Design review of the part built by this model. Coordinates are the model's own, in mm. A direction names the side the tool comes from. Round coordinates to 2 decimals unless told otherwise and drop trailing zeros. Write each loop counter-clockwise with the first axis right and the second up, starting at its lowest first coordinate (ties: lowest second). Pieces come first, ordered by that corner, then holes. Notation, with made-up numbers: (-31, 78.25) - (-13, 78.25) arc R24 cw to (-13, 113.25) - close; hole circle Ø11 at (58.25, 20). An arc over 180 degrees is marked (long way). Use one line per item in the form item = value.
```python
from build123d import *

# Parameters (mm, degrees)
EXTRUSION1_DEPTH = 100
EXTRUSION2_DEPTH = 100
EXTRUSION3_DEPTH = 100
EXTRUSION4_DEPTH = 200
EXTRUSION5_DEPTH = 10
ESQUISSE6_R      = 40
EXTRUSION6_DEPTH = 300
ESQUISSE7_W      = 3
ESQUISSE7_H      = 195
EXTRUSION8_DEPTH = 250
CONG_1_R         = 50
ESQUISSE8_W      = 3
ESQUISSE8_H      = 150
EXTRUSION9_DEPTH = 0.5


with BuildPart() as part:
    # Esquisse1 → Extrusion1 (new body)
    with BuildSketch(Plane(origin=(0, 0, 0), x_dir=(1, 0, 0), z_dir=(0, 1, 0))):
        with BuildLine():
            Line((-500, 0), (0, 0))
            Line((0, 0), (500, 0))
            ThreePointArc((500, 0), (0, -500), (-500, 0))
        make_face()
    extrude(amount=EXTRUSION1_DEPTH)

    # Esquisse2 → Extrusion2 (add)
    with BuildSketch(Plane(origin=(0, 100, 0), x_dir=(-1, 0, 0), z_dir=(0, 1, 0))):
        with BuildLine():
            Line((400, 0), (-400, 0))
            ThreePointArc((-400, 0), (0, 400), (400, 0))
        make_face()
    extrude(amount=EXTRUSION2_DEPTH)

    # Esquisse3 → Extrusion3 (add)
    with BuildSketch(Plane(origin=(0, 200, 0), x_dir=(-1, 0, 0), z_dir=(0, 1, 0))):
        with BuildLine():
            Line((300, 0), (-300, 0))
            ThreePointArc((-300, 0), (0, 300), (300, 0))
        make_face()
    extrude(amount=EXTRUSION3_DEPTH)

    # Esquisse4 → Extrusion4 (add)
    with BuildSketch(Plane(origin=(0, 300, 0), x_dir=(-1, 0, 0), z_dir=(0, 1, 0))):
        with BuildLine():
            Line((200, 0), (197, 0))
            ThreePointArc((197, 0), (0, 197), (-197, 0))
            Line((-197, 0), (-200, 0))
            ThreePointArc((-200, 0), (0, 200), (200, 0))
        make_face()
    extrude(amount=EXTRUSION4_DEPTH)

    # Esquisse5 → Extrusion5 (add)
    with BuildSketch(Plane(origin=(0, 0, 0), x_dir=(-1, 0, 0), z_dir=(0, 0, -1))):
        with BuildLine():
            Line((200, 700), (-200, 700))
            Line((-200, 700), (-200, 300))
            Line((-200, 300), (-300, 300))
            Line((-300, 300), (-300, 200))
            Line((-300, 200), (-400, 200))
            Line((-400, 200), (-400, 100))
            Line((-400, 100), (-500, 100))
            Line((-500, 100), (-500, 70))
            Line((-500, 70), (-305.941170816, 70))
            ThreePointArc((-305.941170816, 70), (0, 250), (305.941170816, 70))
            Line((305.941170816, 70), (500, 70))
            Line((500, 70), (500, 100))
            Line((500, 100), (400, 100))
            Line((400, 100), (400, 200))
            Line((400, 200), (300, 200))
            Line((300, 200), (300, 300))
            Line((300, 300), (200, 300))
            Line((200, 300), (200, 700))
        make_face()
    extrude(amount=EXTRUSION5_DEPTH)

    # Esquisse6 → Extrusion6 (cut)
    with BuildSketch(Plane(origin=(0, 300, 0), x_dir=(1, 0, 0), z_dir=(0, 1, 0))):
        with Locations((-343.274848141, -68.281612706)):
            Circle(ESQUISSE6_R)
        with Locations((-291.014364306, -194.449581557)):
            Circle(ESQUISSE6_R)
        with Locations((-446.150187618, -58.736786499)):
            Circle(ESQUISSE6_R)
        with Locations((-415.74578963, -172.207544564)):
            Circle(ESQUISSE6_R)
        with Locations((-357.009003131, -273.942643054)):
            Circle(ESQUISSE6_R)
        with Locations((-273.942643054, -357.009003131)):
            Circle(ESQUISSE6_R)
        with Locations((-172.207544564, -415.74578963)):
            Circle(ESQUISSE6_R)
        with Locations((-58.736786499, -446.150187618)):
            Circle(ESQUISSE6_R)
        with Locations((58.736786499, -446.150187618)):
            Circle(ESQUISSE6_R)
        with Locations((172.207544564, -415.74578963)):
            Circle(ESQUISSE6_R)
        with Locations((273.942643054, -357.009003131)):
            Circle(ESQUISSE6_R)
        with Locations((357.009003131, -273.942643054)):
            Circle(ESQUISSE6_R)
        with Locations((415.74578963, -172.207544564)):
            Circle(ESQUISSE6_R)
        with Locations((446.150187618, -58.736786499)):
            Circle(ESQUISSE6_R)
        with Locations((-194.449581557, -291.014364306)):
            Circle(ESQUISSE6_R)
        with Locations((-68.281612706, -343.274848141)):
            Circle(ESQUISSE6_R)
        with Locations((68.281612706, -343.274848141)):
            Circle(ESQUISSE6_R)
        with Locations((194.449581557, -291.014364306)):
            Circle(ESQUISSE6_R)
        with Locations((291.014364306, -194.449581557)):
            Circle(ESQUISSE6_R)
        with Locations((343.274848141, -68.281612706)):
            Circle(ESQUISSE6_R)
    extrude(amount=-EXTRUSION6_DEPTH, mode=Mode.SUBTRACT)

    # Esquisse7 → Extrusion8 (add)
    with BuildSketch(Plane(origin=(0, 300, 0), x_dir=(1, 0, 0), z_dir=(0, 1, 0))):
        with Locations((0, -97.5)):
            Rectangle(ESQUISSE7_W, ESQUISSE7_H)
    extrude(amount=EXTRUSION8_DEPTH)

    # Congé1
    cong_1_edges = [part.edges().sort_by_distance(p)[0] for p in [
        (0, 550, 195),
    ]]
    fillet(cong_1_edges, radius=CONG_1_R)

    # Esquisse8 → Extrusion9 (cut)
    with BuildSketch(Plane.XY):
        with Locations((0, 625)):
            Rectangle(ESQUISSE8_W, ESQUISSE8_H)
    extrude(amount=-EXTRUSION9_DEPTH, mode=Mode.SUBTRACT)


solid = part.part
```
Q1. We need section A-A on y = 570. Write out the cut boundary in (x, z), then the cut area to 3 significant figures.
Calculated:
outline = (-200, -10) - (200, -10) - (200, 0) - (1.5, 0) - (1.5, -0.5) - (-1.5, -0.5) - (-1.5, 0) - (-200, 0) - close
area = 4,000 mm2
Q2. To check wall thickness, follow line 1 along X through (y, z) = (72, 197); line 2 along X through (y, z) = (476, 59); line 3 along Z through (x, y) = (-223, 43). State the ranges of each line that lie inside material, in increasing order. Write a range as from..to.
Calculated:
line_1 = -459.56..-447.14, -384.36..-330.93, -251.1..251.1, 330.93..384.36, 447.14..459.56
line_2 = -191.1..-187.96, -1.5..1.5, 187.96..191.1
line_3 = 0..263, 319.03..447.52
Q3. Draft analysis for pull direction X (two halves, no side actions). For faces 4 (the flat face through (7, 0, 247)), 5 (the cylindrical face through (-4.332, 398.6, 196.952)), 6 (the cylindrical face through (4.4, 398.6, 199.95)), state which applies: released by +X, released by -X, zero draft, split by the parting line, or undercut.
Calculated:
face_4 = zero draft
face_5 = undercut
face_6 = split by the parting line
Q4. We need section B-B on x = -78.5. Write out the cut boundary in (y, z), then the cut area to 3 significant figures.
Calculated:
outline = (0, 0) - (241.08, 0) - (241.08, -10) - (700, -10) - (700, 0) - (300, 0) - (300, 180.68) - (500, 180.68) - (500, 183.95) - (300, 183.95) - (300, 289.55) - (200, 289.55) - (200, 304.6) - (0, 304.6) - close; (0, 381.95) - (200, 381.95) - (200, 392.22) - (100, 392.22) - (100, 411.37) - (0, 411.37) - close; (0, 480.93) - (100, 480.93) - (100, 493.8) - (0, 493.8) - close
area = 100,000 mm2
Q5. We need section C-C on y = 115.5. State how many separate pieces and enclosed holes the cut face has, then the cut area to 3 significant figures.
Calculated:
separate_pieces = 1
enclosed_holes = 8
area = 214,000 mm2
Q6. We need section D-D on x = 343. Write out the cut boundary in (y, z), then the cut area to 3 significant figures.
Calculated:
outline = (0, 0) - (70, 0) - (70, -10) - (200, -10) - (200, 28.28) - (0, 28.28) - close; (0, 108.28) - (200, 108.28) - (200, 205.79) - (100, 205.79) - (100, 236.48) - (0, 236.48) - close; (0, 311.41) - (100, 311.41) - (100, 363.8) - (0, 363.8) - close
area = 34,800 mm2
Q7. For P1, Ø12, axis at x = -266.5, z = 275, coming from the +Y side; P2, Ø8, axis at y = 462.5, z = 153.5, coming from the -X side; P3, Ø5, axis at y = 171.5, z = -5.5, coming from the +X side; P4, Ø2, axis at x = -383, z = 134.5, coming from the -Y side, all flat-tipped, find the tip position at first contact; note any pin that passes through.
Calculated:
P1 = 200
P2 = -132.85
P3 = 400
P4 = 0
Q8. Machinability: for faces 1 (the cylindrical face through (5.21, 249.96, -4.93)), 2 (the flat face through (-2, 200, 302)), 3 (the flat face through (102, 503, 0)), which of the approach directions +Z, -Z, +X, -X, +Y, -Y give a long, thin tool a straight path to every point of the face, cutting with its end or side? Answer none if there is none.
Calculated:
face_1 = -Z, -Y
face_2 = +Z, +Y
face_3 = +Y
